```python
from build123d import *

# Parameters (mm, degrees)
SKETCH1_W           = 28
SKETCH1_H           = 142
BOSS_EXTRUDE1_DEPTH = 4
BOSS_EXTRUDE2_DEPTH = 35
SKETCH1_5_W         = 28
SKETCH1_5_H         = 2
BOSS_EXTRUDE3_DEPTH = 17.5
CUT_EXTRUDE1_REACH  = 82.907
SKETCH2_R           = 1.7
SKETCH2_3_R         = 3.05
CUT_EXTRUDE2_DEPTH  = 2
CUT_EXTRUDE3_DEPTH  = 88.051708771


with BuildPart() as part:
    # Sketch1 → Boss-Extrude1 (new body)
    with BuildSketch(Plane(origin=(0, 0, 0), x_dir=(1, 0, 0), z_dir=(0, 1, 0))):
        Rectangle(SKETCH1_W, SKETCH1_H)
    extrude(amount=BOSS_EXTRUDE1_DEPTH)

    # Sketch1_4 → Boss-Extrude2 (add)
    with BuildSketch(Plane(origin=(0, 0, 0), x_dir=(1, 0, 0), z_dir=(0, 1, 0))):
        Polygon((-14, -73), (-14, -71), (-14, 71), (14, 71), (14, -71), (14, -73), (16, -73), (16, 73), (-16, 73), (-16, -73), align=None)
    extrude(amount=BOSS_EXTRUDE2_DEPTH)

    # Sketch1_5 → Boss-Extrude3 (add)
    with BuildSketch(Plane(origin=(0, 0, 0), x_dir=(1, 0, 0), z_dir=(0, 1, 0))):
        with Locations((0, -72)):
            Rectangle(SKETCH1_5_W, SKETCH1_5_H)
    extrude(amount=BOSS_EXTRUDE3_DEPTH)

    # Sketch2 → Cut-Extrude1 (cut, up to next)
    with BuildSketch(Plane(origin=(0, 4, 0), x_dir=(1, 0, 0), z_dir=(0, 1, 0)), mode=Mode.PRIVATE) as cut_extrude1_sk1:
        with Locations(Location((0, 30, 0), (0, 0, 270))):
            Circle(SKETCH2_R)
    cut_extrude1_tool1 = extrude(cut_extrude1_sk1.sketch, amount=-CUT_EXTRUDE1_REACH, mode=Mode.PRIVATE) & part.part
    # Sketch2 → Cut-Extrude1 (cut, up to next)
    with BuildSketch(Plane(origin=(0, 4, 0), x_dir=(1, 0, 0), z_dir=(0, 1, 0)), mode=Mode.PRIVATE) as cut_extrude1_sk2:
        with Locations(Location((0, -30, 0), (0, 0, 270))):
            Circle(SKETCH2_R)
    cut_extrude1_tool2 = extrude(cut_extrude1_sk2.sketch, amount=-CUT_EXTRUDE1_REACH, mode=Mode.PRIVATE) & part.part
    add(cut_extrude1_tool1.solids().sort_by_distance((0, 4, -30))[0], mode=Mode.SUBTRACT)
    add(cut_extrude1_tool2.solids().sort_by_distance((0, 4, 30))[0], mode=Mode.SUBTRACT)

    # Sketch2_3 → Cut-Extrude2 (cut)
    with BuildSketch(Plane(origin=(0, 4, 0), x_dir=(1, 0, 0), z_dir=(0, 1, 0))):
        with Locations(Location((0, 30, 0), (0, 0, 270))):
            Circle(SKETCH2_3_R)
        with Locations(Location((0, -30, 0), (0, 0, 270))):
            Circle(SKETCH2_3_R)
    extrude(amount=-CUT_EXTRUDE2_DEPTH, mode=Mode.SUBTRACT)

    # Sketch3 → Cut-Extrude3 (cut, through all)
    with BuildSketch(Plane(origin=(16, 0, 0), x_dir=(0, 0, -1), z_dir=(1, 0, 0))):
        Polygon((-73, 17.5), (-55.5, 35), (-73, 35), align=None)
    extrude(amount=-CUT_EXTRUDE3_DEPTH, mode=Mode.SUBTRACT)


solid = part.part
```
Could you check a few things on this model? Use its own coordinates, in mm. A direction names the side the tool comes from. Give positions to 0.01 mm unless a question says otherwise; leave off trailing zeros. Loops run counter-clockwise (first coordinate to the right, second up) from the corner with the lowest first, then second, coordinate; pieces in that order, holes last. Notation, with made-up numbers: (16, 41) - (70, 41) arc R20 ccw to (70, 62) - close; hole circle Ø10 at (-1, 1). An arc over 180 degrees is marked (long way). Use one line per item in the form item = value.
1. I want a section at B-B (z = 30). Please give me the cut outline in (x, y).
Response values:
outline = (-16, 0) - (-1.7, 0) - (-1.7, 2) - (-3.05, 2) - (-3.05, 4) - (-14, 4) - (-14, 35) - (-16, 35) - close; (1.7, 0) - (16, 0) - (16, 35) - (14, 35) - (14, 4) - (3.05, 4) - (3.05, 2) - (1.7, 2) - close
2. I need wall thicknesses on probe 1 along X at (y, z) = (27, 11.5); probe 2 along Z at (x, y) = (-1, 16.5); probe 3 along Y at (x, z) = (3.5, 8). Which ranges of each line are inside material? Lowest first, please.
Response values:
probe_1 = -16 to -14, 14 to 16
probe_2 = -73 to -71, 71 to 73
probe_3 = 0 to 4
3. I'm going to push flat-ended pins straight in: pin 1 Ø3 at (x, z) = (1, -31) entering from +Y; pin 2 Ø4 at (x, z) = (0, -30) entering from -Y; pin 3 Ø2 at (x, z) = (-2.5, 35.5) entering from +Y; pin 4 Ø2 at (x, z) = (5, 72) entering from +Y. Where does each tip first touch, or does it pass through?
Response values:
pin_1 = 2
pin_2 = 0
pin_3 = 4
pin_4 = 17.5
4. On a 3-axis mill with a long thin cutter (end or side, diameter ignored), from which of +Z, -Z, +X, -X, +Y, -Y can I reach the whole of each face in a straight line? I mean faces 4 (the face through (-0.65, 1.01, -28.43)), 5 (the face through (-1.31, 2, 31.31)). Say none if no direction works.
Response values:
face_4 = +Y, -Y
face_5 = +Y
5. I want a section at D-D (y = 23). Please give me the cut outline in (x, z), and give its area (3 significant figures).
Response values:
outline = (-16, -73) - (16, -73) - (16, 67.5) - (14, 67.5) - (14, -71) - (-14, -71) - (-14, 67.5) - (-16, 67.5) - close
area = 618 mm²
6. I want a section at A-A (x = 0). Please give me the cut outline in (y, z).
Response values:
outline = (0, -73) - (35, -73) - (35, -71) - (4, -71) - (4, -33.05) - (2, -33.05) - (2, -31.7) - (0, -31.7) - close; (0, -28.3) - (2, -28.3) - (2, -26.95) - (4, -26.95) - (4, 26.95) - (2, 26.95) - (2, 28.3) - (0, 28.3) - close; (0, 31.7) - (2, 31.7) - (2, 33.05) - (4, 33.05) - (4, 71) - (17.5, 71) - (17.5, 73) - (0, 73) - close
7. I want a section at C-C (z = -19.5). Please give me the cut outline in (x, y), and give its area (3 significant figures).
Response values:
outline = (-16, 0) - (16, 0) - (16, 35) - (14, 35) - (14, 4) - (-14, 4) - (-14, 35) - (-16, 35) - close
area = 252 mm²
8. Thinking about a two-plate mould opening in X: for faces 1 (the face through (0, 0, -1)), 2 (the face through (16, 17, 1)), 3 (the face through (-0.65, 1.01, 31.57)), which applies, released by +X, released by -X, zero draft, split by the parting line, or undercut?
Response values:
face_1 = zero draft
face_2 = released by +X
face_3 = undercut
